The drawing under review shows one solid part. Ordinate dimensions are in mm from its lowest x, y, z. A direction names the side the tool comes from. Coordinates: 2 decimals unless noted, no trailing zeros. Order: outer loops, then holes, each group sorted by start corner. A loop starts at its lowest first (then second) coordinate and runs counter-clockwise, first axis right, second up. Notation, with made-up numbers: (-27, -18) -> (25, -18) arc R28 ccw to (25, 19) -> close; hole circle Ø11 at (-31, -5). An arc over 180 degrees is marked (long way). Put each result on its own line as item: value.
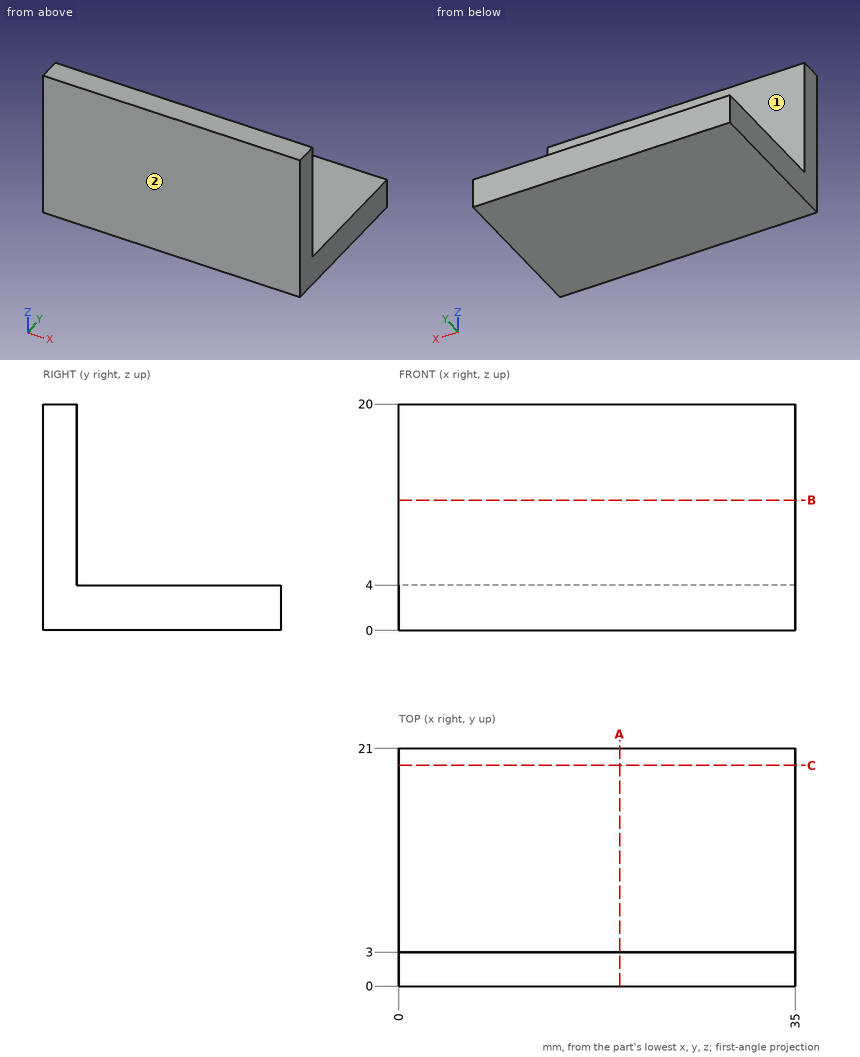
Item 1: Consider section C-C on y = 19.5. Write out the cut boundary in (x, z), and give its area (3 significant figures).
Answers below:
outline: (0, 0) -> (35, 0) -> (35, 4) -> (0, 4) -> close
area: 140 mm^2
Item 2: For line 1 (Y direction, x = 32, z = 17); line 2 (Z direction, x = 5.5, y = 4), list the stretches that pass through material, from the lowest coordinate up. Write a range as from..to.
Answers below:
line 1: 0..3
line 2: 0..4
Item 3: Consider section A-A on x = 19.5. Write out the cut boundary in (y, z), and give its area (3 significant figures).
Answers below:
outline: (0, 0) -> (21, 0) -> (21, 4) -> (3, 4) -> (3, 20) -> (0, 20) -> close
area: 132 mm^2
Item 4: For pin 1 Ø5.5 at (x, y) = (14.5, 10.5) entering from +Z; pin 2 Ø8 at (x, z) = (18.5, 11) entering from +Y, all flat-tipped, find the tip position at first contact; note any pin that passes through.
Answers below:
pin 1: z = 4
pin 2: y = 3
Item 5: Consider section B-B on z = 11.5. Write out the cut boundary in (x, y), and give its area (3 significant figures).
Answers below:
outline: (0, 0) -> (35, 0) -> (35, 3) -> (0, 3) -> close
area: 105 mm^2
Item 6: For the marked faces 1 and 2, list the 3-axis set-ups (+Z, -Z, +X, -X, +Y, -Y) from which the entire face can be reached by the end or side of a thin tool; tool diameter is ignored.
Answers below:
face 1: +Z, +X, -X, +Y
face 2: +Z, -Z, +X, -X, -Y
